Can you work these out from the model? Positions are in its coordinate system, mm. Coordinates: 2 decimals unless noted, no trailing zeros. Loops run counter-clockwise (first coordinate to the right, second up) from the corner with the lowest first, then second, coordinate; pieces in that order, holes last.
Autodesk Inventor part; units mm, degrees
ref_plane "Work Plane1" through (0, 0, 0) normal (0, 0, 1) x (1, 0, 0)
ref_plane "YZ Plane" through (0, 0, 0) normal (1, 0, 0) x (0, 1, 0)
ref_plane "XZ Plane" through (0, 0, 0) normal (0, 1, 0) x (-1, 0, 0)
ref_plane "Work Plane1" through (0, 0, 0) normal (0, 0, 1) x (1, 0, 0)
sketch "Sketch1" plane through (0, 0, 0) normal (0, 0, 1) x (1, 0, 0)
  line L0 (0, 0) -> (0, -96.52)
  line L1 (0, -96.52) -> (25.4, -96.52)
  line L2 (25.4, -96.52) -> (53.34, -80.3888)
  arc A0 (53.34, -80.3888) -> (57.7429, -57.8254) centre (45.72, -67.1906) ccw
  line L3 (57.7429, -57.8254) -> (12.7, 0)
  line L4 (12.7, 0) -> (0, 0)
  dimension "d0" = 96.52
  dimension "d1" = 25.4
  dimension "d2" = 60.96
  dimension "d3" = 15.24
  dimension "d4" = 12.7
  dimension "d5" = 30
extrude "Extrusion1" add sketch "Sketch1" along normal mid plane 12.7
sketch "Sketch2" plane through (0, 0, 6.35) normal (0, 0, 1) x (1, 0, 0)
  arc A0 (53.34, -80.3888) -> (57.7429, -57.8254) centre (45.72, -67.1906) ccw
  point P0 (0, 0)
hole "Hole1" at (45.72, -67.1906, 6.35) direction (0, 0, -1) diameter 13.8938 end through all
properties part number "Catch plate"
(1) I want a section at B-B on y = -64. Write out the boundary of the cut face in (x, z).
Check values:
outline: (0, -6.35) - (39.55, -6.35) - (39.55, 6.35) - (0, 6.35) - close; (51.89, -6.35) - (60.62, -6.35) - (60.62, 6.35) - (51.89, 6.35) - close
(2) I want a section at D-D on y = -48. Write out the boundary of the cut face in (x, z).
Check values:
outline: (0, -6.35) - (50.09, -6.35) - (50.09, 6.35) - (0, 6.35) - close
(3) If I drill on probe 1 along X at (y, z) = (-67, 3.25); probe 2 along X at (y, z) = (-71.5, -0.5); probe 3 along Y at (x, z) = (52, 5.5), over which ranges is the centre line in solid material (lowest first)?
Check values:
probe 1: x = 0 to 38.78, 52.66 to 60.96
probe 2: x = 0 to 40.27, 51.17 to 60.34
probe 3: y = -81.16 to -70.16, -64.22 to -50.45
(4) I want a section at C-C on x = 45.72. Write out the boundary of the cut face in (y, z), then the cut area to 3 significant figures.
Check values:
outline: (-84.79, -6.35) - (-74.14, -6.35) - (-74.14, 6.35) - (-84.79, 6.35) - close; (-60.24, -6.35) - (-42.39, -6.35) - (-42.39, 6.35) - (-60.24, 6.35) - close
area: 362 mm2
(5) I want a section at A-A on z = 1. Write out the boundary of the cut face in (x, y).
Check values:
outline: (0, -96.52) - (25.4, -96.52) - (53.34, -80.39) arc R15.24 ccw to (57.74, -57.83) - (12.7, 0) - (0, 0) - close; hole circle Ø13.89 at (45.72, -67.19)
(6) If we mould it in two halves opening along X, with no side actions, what happens to faces 1 (the cylindrical face through (38.83, -66.29, -0.09)), 2 (the flat face through (6, 0, 0)), 3 (the flat face through (39.17, -88.57, -0.09))? For each: released by +X, released by -X, zero draft, split by the parting line, or undercut.
Check values:
face 1: undercut
face 2: zero draft
face 3: released by +X
(7) I'm going to push a flat-ended pin straight in: pin 1 (1 mm diameter, centred on x = 15.5, z = -1.5, fed in from +Y). Where does the tip first touch, or does it pass through?
Check values:
pin 1: stops at y = -2.95
